For this review, take the finished solid that the model builds, in its own axes (mm). A direction names the side the tool comes from. Give positions to 0.01 mm unless a question says otherwise; leave off trailing zeros. Order: outer loops, then holes, each group sorted by start corner. A loop starts at its lowest first (then second) coordinate and runs counter-clockwise, first axis right, second up. Notation, with made-up numbers: (28, -8.5) -> (69, -8.5) arc R22 cw to (69, 2.5) -> close; hole circle Ø7 at (-8, 44.25). An arc over 180 degrees is marked (long way). Return JSON: item names as keys, results as strings. Group by question number.
1) For faces 4 (the face through (-415, -12, 317.5)), 5 (the face through (202.047, 162, 272)), 6 (the face through (-408.329, -2, 121)), list the 3-axis set-ups (+Z, -Z, +X, -X, +Y, -Y) from which the entire face can be reached by the end or side of a thin tool; tool diameter is ignored.
2) Add section D-D (y = 0). Give the boundary of the cut face in (x, z).
3) The part is to be moulded in two halves that separate along X. For faces 1 (the face through (-3, 162, 228.202)), 2 (the face through (426.98, -26.46, 151.19)), 3 (the face through (-446.162, -2, 121)), say which applies: released by +X, released by -X, zero draft, split by the parting line, or undercut.
4) To check wall thickness, follow line 1 along Y through (x, z) = (-346.5, 64); line 2 along Z through (x, y) = (426.5, 0); line 3 along X through (y, z) = (120.5, 141). State the ranges of each line that lie inside material, in increasing order.
5) Add section B-B (z = 98). Give the boundary of the cut face in (x, y), then the cut area to 3 significant figures.
6) Add section C-C (x = 171.5). Give the boundary of the cut face in (y, z).
7) Add section A-A (y = -98). Give the boundary of the cut face in (x, z), then the cut area to 3 significant figures.
8) Insertion check: P1, Ø9.5, axis at x = 12.5, y = 162.5, coming from the +Z side. The pin has a flat end and moves straight along its axis. Give the tip position at first contact, or say it passes through.
from build123d import *

# Parameters (mm, degrees)
F0_W     = 892.323136
F0_H     = 355.258762
F0_W_2   = 816.658438
F0_H_2   = 292.204798
F1_DEPTH = 317.5
F2_W     = 404.093236
F2_H     = 178.596606
F3_DEPTH = 355.259763
F4_R     = 57.353044
F5_DEPTH = 892.324136


with BuildPart() as f1:
    # F0 (on Top) → F1 (new body)
    with BuildSketch(Plane.XY):
        Rectangle(F0_W, F0_H)
        Rectangle(F0_W_2, F0_H_2, mode=Mode.SUBTRACT)
    extrude(amount=F1_DEPTH)

    # F2 (on face) → F3 (cut, through all)
    with BuildSketch(Plane.XZ.offset(177.629381)):
        with Locations((0, 317.5)):
            Rectangle(F2_W, F2_H)
    extrude(amount=-F3_DEPTH, mode=Mode.SUBTRACT)

    # F4 (on face) → F5 (cut, through all)
    with BuildSketch(Plane(origin=(-446.161568, 0, 0), x_dir=(0, -1, 0), z_dir=(-1, 0, 0))):
        with Locations((0, 202.074319)):
            Circle(F4_R)
    extrude(amount=-F5_DEPTH, mode=Mode.SUBTRACT)


solid = f1.part
Evaluation:
{
 "1": {"face 4": "+Z, +X, -X, +Y, -Y", "face 5": "+Z, +Y, -Y", "face 6": "+Z, -Z"},
 "2": {"outline": "(-446.16, 0) -> (-408.33, 0) -> (-408.33, 144.72) -> (-446.16, 144.72) -> close; (-446.16, 259.43) -> (-408.33, 259.43) -> (-408.33, 317.5) -> (-446.16, 317.5) -> close; (408.33, 0) -> (446.16, 0) -> (446.16, 144.72) -> (408.33, 144.72) -> close; (408.33, 259.43) -> (446.16, 259.43) -> (446.16, 317.5) -> (408.33, 317.5) -> close"},
 "3": {"face 1": "undercut", "face 2": "zero draft", "face 3": "released by -X"},
 "4": {"line 1": "-177.63 to -146.1, 146.1 to 177.63", "line 2": "0 to 144.72, 259.43 to 317.5", "line 3": "-446.16 to -408.33, 408.33 to 446.16"},
 "5": {"outline": "(-446.16, -177.63) -> (446.16, -177.63) -> (446.16, 177.63) -> (-446.16, 177.63) -> close; hole (-408.33, -146.1) -> (408.33, -146.1) -> (408.33, 146.1) -> (-408.33, 146.1) -> close", "area": "78,400 mm^2"},
 "6": {"outline": "(-177.63, 0) -> (-146.1, 0) -> (-146.1, 228.2) -> (-177.63, 228.2) -> close; (146.1, 0) -> (177.63, 0) -> (177.63, 228.2) -> (146.1, 228.2) -> close"},
 "7": {"outline": "(-446.16, 0) -> (-408.33, 0) -> (-408.33, 317.5) -> (-446.16, 317.5) -> close; (408.33, 0) -> (446.16, 0) -> (446.16, 317.5) -> (408.33, 317.5) -> close", "area": "24,000 mm^2"},
 "8": {"P1": "z = 228.2"}
}
